```python
from build123d import *

# Parameters (mm, degrees)
F1_DEPTH = 3.175
F2_W     = 111.125
F2_H     = 1.5875
F3_DEPTH = 15.875
F4_W     = 111.125
F4_H     = 19.05
F5_DEPTH = 1.5748
F6_W     = 111.125
F6_H     = 3.1623
F7_DEPTH = 25.4


with BuildPart() as f1:
    # F0 (on Front) → F1 (new body)
    with BuildSketch(Plane.XZ):
        with BuildLine():
            ThreePointArc((0, -6.35), (-4.4901280605, -4.4901280605), (-6.35, 0))
            Line((-6.35, 0), (-7.9375, 0))
            ThreePointArc((-7.9375, 0), (-5.6126600757, -5.6126600757), (0, -7.9375))
            Line((0, -7.9375), (0, -6.35))
        make_face()
        with BuildLine():
            Line((-7.9375, 0), (-6.35, 0))
            ThreePointArc((-6.35, 0), (0, 6.35), (6.35, 0))
            Line((6.35, 0), (7.9375, 0))
            ThreePointArc((7.9375, 0), (0, 7.9375), (-7.9375, 0))
        make_face()
        with BuildLine():
            Line((7.9375, 0), (6.35, 0))
            ThreePointArc((6.35, 0), (4.4901280605, -4.4901280605), (0, -6.35))
            Line((0, -6.35), (0, -7.9375))
            ThreePointArc((0, -7.9375), (5.6126600757, -5.6126600757), (7.9375, 0))
        make_face()
        with BuildLine():
            ThreePointArc((0, -7.9375), (-5.6126600757, -5.6126600757), (-7.9375, 0))
            Line((-7.9375, 0), (-11.1125, 0))
            ThreePointArc((-11.1125, 0), (-13.4373399347, -5.6126600861), (-19.0500000294, -7.9375))
            Line((-19.0500000294, -7.9375), (0, -7.9375))
        make_face()
        with BuildLine():
            Line((7.9375, -7.9375), (7.9375, 0))
            ThreePointArc((7.9375, 0), (5.6126600757, -5.6126600757), (0, -7.9375))
            Line((0, -7.9375), (7.9375, -7.9375))
        make_face()
        Polygon((7.9375, -7.9375), (0, -7.9375), (-19.0500000294, -7.9375), (-38.1000000951, -7.9375), (-57.15, -7.9375), (-76.2, -7.9375), (-95.25, -7.9375), (-103.1875, -7.9375), (-103.1875, -9.525), (7.9375, -9.525), align=None)
        with BuildLine():
            ThreePointArc((-19.0500000294, -7.9375), (-13.4373399347, -5.6126600861), (-11.1125, 0))
            Line((-11.1125, 0), (-12.7, 0))
            ThreePointArc((-12.7, 0), (-19.05, -6.35), (-25.4, 0))
            Line((-25.4, 0), (-26.9875, 0))
            ThreePointArc((-26.9875, 0), (-24.6626600861, -5.6126600653), (-19.0500000294, -7.9375))
        make_face()
        with BuildLine():
            Line((-12.7, 0), (-11.1125, 0))
            ThreePointArc((-11.1125, 0), (-19.05, 7.9375), (-26.9875, 0))
            Line((-26.9875, 0), (-25.4, 0))
            ThreePointArc((-25.4, 0), (-19.05, 6.35), (-12.7, 0))
        make_face()
        with BuildLine():
            Line((-38.1000000951, -7.9375), (-19.0500000294, -7.9375))
            ThreePointArc((-19.0500000294, -7.9375), (-24.6626600861, -5.6126600653), (-26.9875, 0))
            Line((-26.9875, 0), (-30.1625, 0))
            ThreePointArc((-30.1625, 0), (-32.487339958, -5.6126601093), (-38.1000000951, -7.9375))
        make_face()
        with BuildLine():
            Line((-57.15, -7.9375), (-38.1000000951, -7.9375))
            ThreePointArc((-38.1000000951, -7.9375), (-43.7126601093, -5.612660042), (-46.0375, 0))
            Line((-46.0375, 0), (-49.2125, 0))
            ThreePointArc((-49.2125, 0), (-51.5373399243, -5.6126600757), (-57.15, -7.9375))
        make_face()
        with BuildLine():
            ThreePointArc((-46.0375, 0), (-43.7126601093, -5.612660042), (-38.1000000951, -7.9375))
            ThreePointArc((-38.1000000951, -7.9375), (-32.487339958, -5.6126601093), (-30.1625, 0))
            Line((-30.1625, 0), (-31.75, 0))
            ThreePointArc((-31.75, 0), (-38.1, -6.35), (-44.45, 0))
            Line((-44.45, 0), (-46.0375, 0))
        make_face()
        with BuildLine():
            Line((-31.75, 0), (-30.1625, 0))
            ThreePointArc((-30.1625, 0), (-38.1, 7.9375), (-46.0375, 0))
            Line((-46.0375, 0), (-44.45, 0))
            ThreePointArc((-44.45, 0), (-38.1, 6.35), (-31.75, 0))
        make_face()
        with BuildLine():
            Line((-76.2, -7.9375), (-57.15, -7.9375))
            ThreePointArc((-57.15, -7.9375), (-62.7626600757, -5.6126600757), (-65.0875, 0))
            Line((-65.0875, 0), (-68.2625, 0))
            ThreePointArc((-68.2625, 0), (-70.5873399243, -5.6126600757), (-76.2, -7.9375))
        make_face()
        with BuildLine():
            ThreePointArc((-65.0875, 0), (-62.7626600757, -5.6126600757), (-57.15, -7.9375))
            ThreePointArc((-57.15, -7.9375), (-51.5373399243, -5.6126600757), (-49.2125, 0))
            Line((-49.2125, 0), (-50.8, 0))
            ThreePointArc((-50.8, 0), (-57.15, -6.35), (-63.5, 0))
            Line((-63.5, 0), (-65.0875, 0))
        make_face()
        with BuildLine():
            Line((-103.1875, 0), (-103.1875, -7.9375))
            Line((-103.1875, -7.9375), (-95.25, -7.9375))
            ThreePointArc((-95.25, -7.9375), (-100.8626600757, -5.6126600757), (-103.1875, 0))
        make_face()
        with BuildLine():
            Line((-50.8, 0), (-49.2125, 0))
            ThreePointArc((-49.2125, 0), (-57.15, 7.9375), (-65.0875, 0))
            Line((-65.0875, 0), (-63.5, 0))
            ThreePointArc((-63.5, 0), (-57.15, 6.35), (-50.8, 0))
        make_face()
        with BuildLine():
            Line((-95.25, -7.9375), (-76.2, -7.9375))
            ThreePointArc((-76.2, -7.9375), (-81.8126600757, -5.6126600757), (-84.1375, 0))
            Line((-84.1375, 0), (-87.3125, 0))
            ThreePointArc((-87.3125, 0), (-89.6373399243, -5.6126600757), (-95.25, -7.9375))
        make_face()
        with BuildLine():
            ThreePointArc((-84.1375, 0), (-81.8126600757, -5.6126600757), (-76.2, -7.9375))
            ThreePointArc((-76.2, -7.9375), (-70.5873399243, -5.6126600757), (-68.2625, 0))
            Line((-68.2625, 0), (-69.85, 0))
            ThreePointArc((-69.85, 0), (-76.2, -6.35), (-82.55, 0))
            Line((-82.55, 0), (-84.1375, 0))
        make_face()
        with BuildLine():
            Line((-101.6, 0), (-103.1875, 0))
            ThreePointArc((-103.1875, 0), (-100.8626600757, -5.6126600757), (-95.25, -7.9375))
            Line((-95.25, -7.9375), (-95.25, -6.35))
            ThreePointArc((-95.25, -6.35), (-99.7401280605, -4.4901280605), (-101.6, 0))
        make_face()
        with BuildLine():
            ThreePointArc((-87.3125, 0), (-95.25, 7.9375), (-103.1875, 0))
            Line((-103.1875, 0), (-101.6, 0))
            ThreePointArc((-101.6, 0), (-95.25, 6.35), (-88.9, 0))
            Line((-88.9, 0), (-87.3125, 0))
        make_face()
        with BuildLine():
            Line((-95.25, -6.35), (-95.25, -7.9375))
            ThreePointArc((-95.25, -7.9375), (-89.6373399243, -5.6126600757), (-87.3125, 0))
            Line((-87.3125, 0), (-88.9, 0))
            ThreePointArc((-88.9, 0), (-90.7598719395, -4.4901280605), (-95.25, -6.35))
        make_face()
        with BuildLine():
            Line((-69.85, 0), (-68.2625, 0))
            ThreePointArc((-68.2625, 0), (-76.2, 7.9375), (-84.1375, 0))
            Line((-84.1375, 0), (-82.55, 0))
            ThreePointArc((-82.55, 0), (-76.2, 6.35), (-69.85, 0))
        make_face()
    extrude(amount=F1_DEPTH)

    # F2 (on face) → F3 (join)
    with BuildSketch(Plane.XZ.offset(3.175)):
        with Locations((-47.625, -8.73125)):
            Rectangle(F2_W, F2_H)
    extrude(amount=F3_DEPTH)

    # F4 (on face) → F5 (join)
    with BuildSketch(Plane(origin=(0, 0, -9.525), x_dir=(1, 0, 0), z_dir=(0, 0, -1))):
        with Locations((-47.625, 9.525)):
            Rectangle(F4_W, F4_H)
    extrude(amount=F5_DEPTH)

    # F6 (on face) → F7 (cut)
    with BuildSketch(Plane.XZ.offset(19.05)):
        with Locations((-47.625, -9.51865)):
            Rectangle(F6_W, F6_H)
    extrude(amount=-F7_DEPTH, mode=Mode.SUBTRACT)


solid = f1.part
```
For this review, take the finished solid that the model builds, in its own axes (mm). A direction names the side the tool comes from. Give positions to 0.01 mm unless a question says otherwise; leave off trailing zeros. Write each loop counter-clockwise with the first axis right and the second up, starting at its lowest first coordinate (ties: lowest second). Pieces come first, ordered by that corner, then holes.
Item 1: Insertion check: P1, Ø1, axis at x = -9.5, y = -1.5, coming from the +Z side; P2, Ø1, axis at x = -52.5, z = 2, coming from the +Y side (3 decimals); P3, Ø1.5, axis at x = -24.5, z = -3, coming from the +Y side. Each pin has a flat end and moves straight along its axis. Give the tip position at first contact, or say it passes through.
Item 2: Take a section at B-B (y = -1.35). Give the number of separate pieces and of enclosed holes in the cut face, and give its area (3 significant figures).
Item 3: Machinability: for faces 5 (the face through (-50.806, -1.565, 0.279)), 6 (the face through (-10, -2, 0)), which of the approach directions +Z, -Z, +X, -X, +Y, -Y give a long, thin tool a straight path to every point of the face, cutting with its end or side? Answer none if there is none.
Item 4: Wall thickness on probe 1 along Z at (x, y) = (-76.2, -2.15); probe 2 along Z at (x, y) = (-15.5, -3): over which ranges is each line inside the solid? List them lowest first.
Item 5: Take a section at D-D (x = -18). Give the boundary of the cut face in (y, z) (1 decimal).
Item 6: The part is to be moulded in two halves that separate along Z. For faces 1 (the face through (-31.756, -1.565, 0.279)), 2 (the face through (0.175, -1.565, 7.936)), 3 (the face through (-48, 0, -2)), 4 (the face through (-48, -2, -7.937)), say which applies: +Z half, -Z half, draft (parallel to the pull), parting line (faces both ways), or undercut.
Established:
1. P1: stops at z = 0
1. P2: passes through
1. P3: stops at y = 0
2. separate pieces: 1
2. enclosed holes: 6
2. area: 716 mm2
3. face 5: +Y, -Y
3. face 6: +Z, +Y, -Y
4. probe 1: z = -7.94 to -6.35, 6.35 to 7.94
4. probe 2: z = -7.94 to -5.26, 5.26 to 7.1
5. outline: (-3.2, -7.9) - (0, -7.9) - (0, -6.3) - (-3.2, -6.3) - close; (-3.2, 6.3) - (0, 6.3) - (0, 7.9) - (-3.2, 7.9) - close
6. face 1: undercut
6. face 2: +Z half
6. face 3: draft
6. face 4: -Z half
